Part print with two shaded views. Sizes in mm from the minimum x, y, z corner. A direction names the side the tool comes from. Coordinates: 2 decimals unless noted, no trailing zeros. Loops run counter-clockwise (first coordinate to the right, second up) from the corner with the lowest first, then second, coordinate; pieces in that order, holes last.
(1) Slice it at C-C (z = 3.5). Give the cut face in (x, y).
(2) Flat gauge pins, fed straight in: P1, Ø4, axis at x = 5, y = 3, coming from the -Z side; P2, Ø4, axis at x = 3.9, y = 3.9, coming from the -Z side; P3, Ø0.8, axis at x = 4.5, z = 15.5, coming from the -Y side (1 decimal); P4, Ø2, axis at x = 6, z = 13.5, coming from the -Y side. Where does each tip first touch, or does it go through?
(3) Slice it at A-A (x = 3.9). Give the cut face in (y, z).
(4) Two-plate mould, pull along Y, no slides. Class the marked faces 1, 2 and 3: pulls with the +Y half, pulls with the -Y half, needs draft (parallel to the pull), parting line crosses it, or undercut.
(5) Slice it at B-B (z = 13.5). Give the cut face in (x, y), and give its area (3 significant figures).
(6) Tool access for the marked faces 4 and 5: list every direction of +Z, -Z, +X, -X, +Y, -Y with a clear straight run to the whole face (end or side of a thin tool).
(7) Wall check: L1, parallel to Y at x = 3.9, z = 13.5; L2, parallel to Y at x = 3.9, z = 6.5; L3, parallel to Z at x = 3, y = 6.25. Give the ranges that are in metal, low to high.
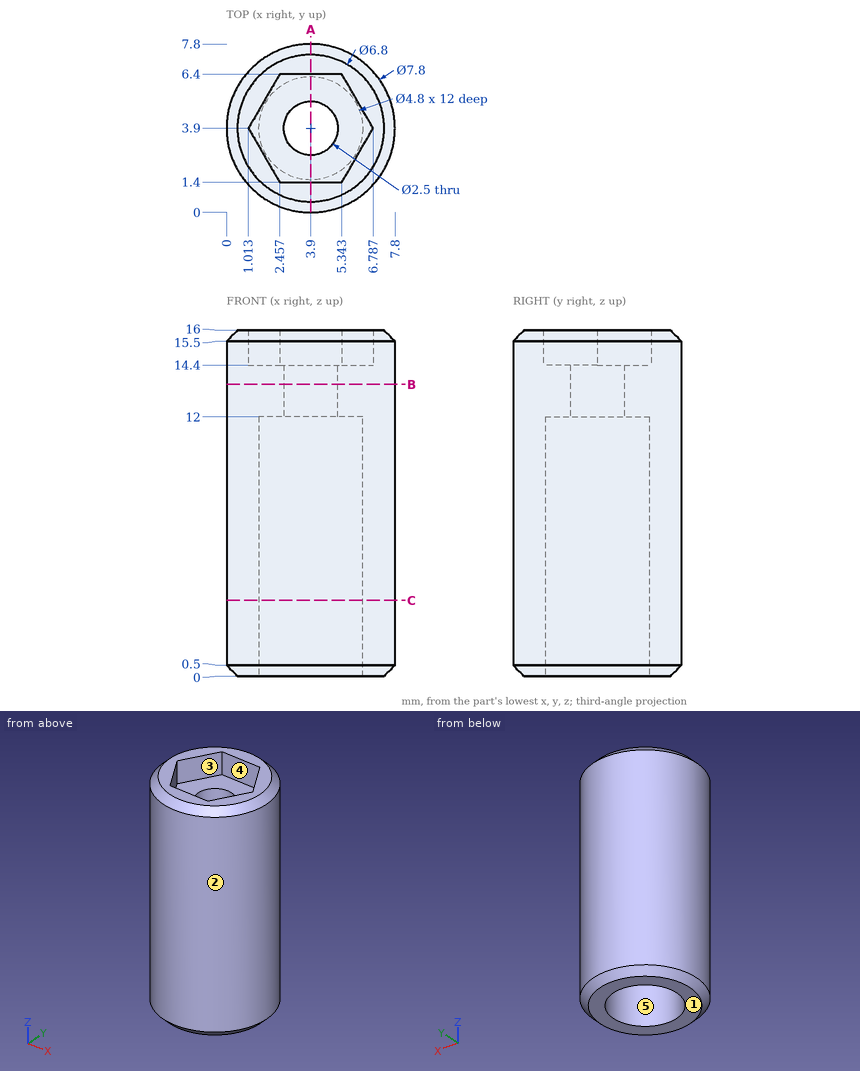
Response values:
1. outline: circle Ø7.8 at (3.9, 3.9); hole circle Ø4.8 at (3.9, 3.9)
2. P1: stops at z = 0
2. P2: stops at z = 12
2. P3: stops at y = 0
2. P4: stops at y = 0.16
3. outline: (0, 0.5) - (0.5, 0) - (1.5, 0) - (1.5, 12) - (2.65, 12) - (2.65, 14.4) - (1.4, 14.4) - (1.4, 16) - (0.5, 16) - (0, 15.5) - close; (5.15, 12) - (6.3, 12) - (6.3, 0) - (7.3, 0) - (7.8, 0.5) - (7.8, 15.5) - (7.3, 16) - (6.4, 16) - (6.4, 14.4) - (5.15, 14.4) - close
4. face 1: needs draft
4. face 2: parting line crosses it
4. face 3: undercut
5. outline: circle Ø7.8 at (3.9, 3.9); hole circle Ø2.5 at (3.9, 3.9)
5. area: 42.9 mm2
6. face 4: +Z
6. face 5: -Z
7. L1: y = 0 to 2.65, 5.15 to 7.8
7. L2: y = 0 to 1.5, 6.3 to 7.8
7. L3: z = 0 to 14.4
